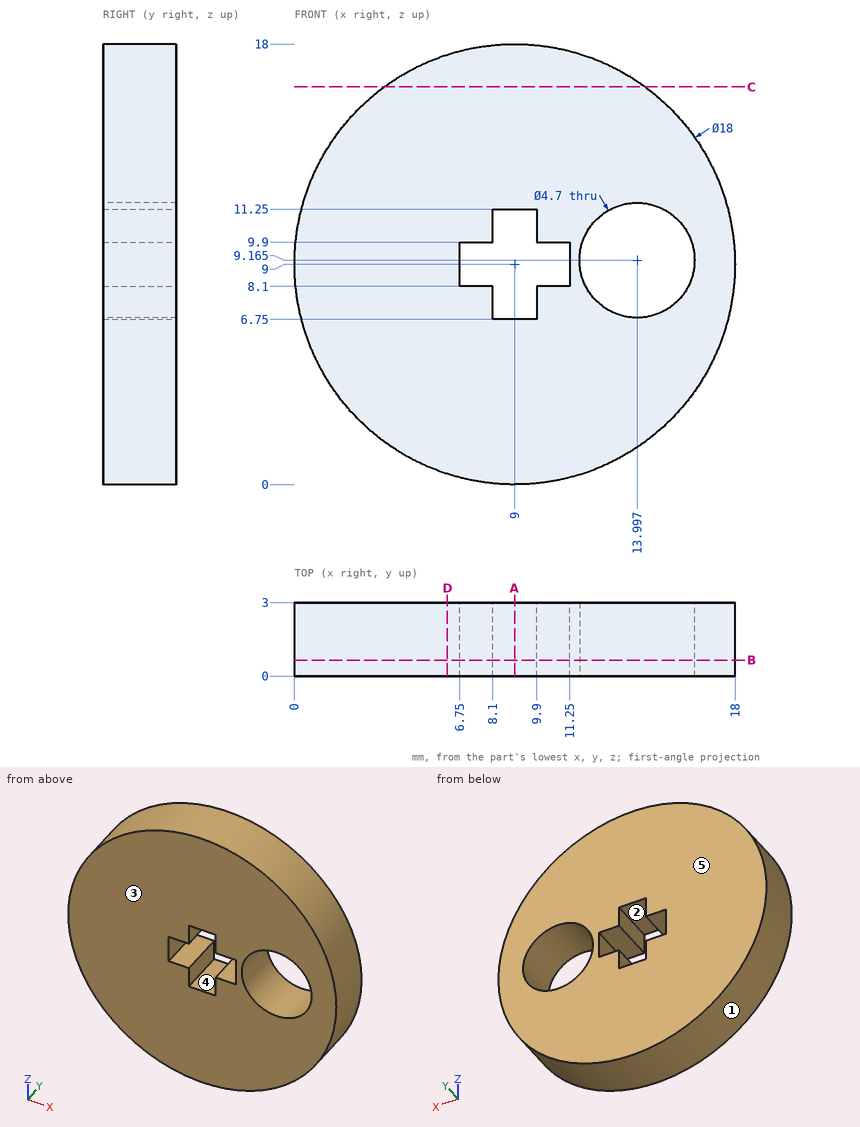
Geometry check sheet. Reference: drawing and pictorial views, mm from the part's lowest x, y, z. A direction names the side the tool comes from. Give positions to 0.01 mm unless a question says otherwise; leave off trailing zeros. Order: outer loops, then holes, each group sorted by start corner. A loop starts at its lowest first (then second) coordinate and runs counter-clockwise, first axis right, second up. Notation, with made-up numbers: M 33,37.25 L 54,37.25 A13 cw 54,41.25 Z; hole C 1.5,89 d6. An arc over 180 degrees is marked long. Return JSON: item names as keys, results as strings. Group by question number.
1) Go/stop test with flat-tipped pins: pin 1 Ø1.5 at (y, z) = (1.5, 12.5) entering from +X; pin 2 Ø1.1 at (x, y) = (10.5, 2) entering from -Z; pin 3 Ø1.1 at (x, y) = (10.5, 1.5) entering from +Z. Record where each tip stops, or that it passes through.
2) Scan lines: line 1 (X direction, y = 2.2, z = 7) (1 decimal); line 2 (X direction, y = 2.8, z = 8.5); line 3 (Z direction, x = 8.75, y = 2.75). Record each from-to range of solid material in increasing order.
3) Section check B-B on y = 0.65. Give the number of separate pieces and of enclosed holes in the cut face, and give its area (3 significant figures).
4) Mould release check, pull along X, two halves, no side actions. Record for the marked faces 1, 2 and 3: pulls with the +X half, pulls with the -X half, needs draft (parallel to the pull), parting line crosses it, or undercut.
5) Section check A-A on x = 9. Record the cut outline in (y, z), and give its area (3 significant figures).
6) Access from +Z, -Z, +X, -X, +Y, -Y to the whole of each face (thin tool, end or side, straight path). Record for the marked faces 4 and 5.
7) Section check D-D on x = 6.25. Record the cut outline in (y, z).
8) Section check C-C on z = 16.25. Record the cut outline in (x, y), and give its area (3 significant figures).
Answer block:
{
 "1": {"pin 1": "stops at x = 17.57", "pin 2": "stops at z = 0.05", "pin 3": "stops at z = 17.95"},
 "2": {"line 1": "x = 0.2 to 8.1, 9.9 to 13.1, 14.9 to 17.8", "line 2": "x = 0.01 to 6.75, 11.25 to 11.74, 16.25 to 17.99", "line 3": "z = 0 to 6.75, 11.25 to 18"},
 "3": {"separate pieces": "1", "enclosed holes": "2", "area": "224 mm^2"},
 "4": {"face 1": "parting line crosses it", "face 2": "undercut", "face 3": "needs draft"},
 "5": {"outline": "M 0,0 L 3,0 L 3,6.75 L 0,6.75 Z; M 0,11.25 L 3,11.25 L 3,18 L 0,18 Z", "area": "40.5 mm^2"},
 "6": {"face 4": "+Y, -Y", "face 5": "+Z, -Z, +X, -X, +Y"},
 "7": {"outline": "M 0,0.43 L 3,0.43 L 3,17.57 L 0,17.57 Z"},
 "8": {"outline": "M 3.67,0 L 14.33,0 L 14.33,3 L 3.67,3 Z", "area": "32.0 mm^2"}
}
